Geometry check sheet. Reference: the model listing, model coordinates, mm. Face numbers are marked on the shaded views. Round coordinates to 2 decimals unless told otherwise and drop trailing zeros. Order: outer loops, then holes, each group sorted by start corner. A loop starts at its lowest first (then second) coordinate and runs counter-clockwise, first axis right, second up. Notation, with made-up numbers: (72, 70) - (89, 70) arc R12 ccw to (89, 81) - close; hole circle Ø2 at (-23.75, -5.5). An arc over 180 degrees is marked (long way). Write each question's results on one line, items separated by ' | '.
```python
from build123d import *

# Parameters (mm, degrees)
SKETCH1_W             = 17.78
SKETCH1_H             = 16.8148
BOSS_EXTRUDE1_DEPTH   = 3.175
SKETCH2_W             = 12.7
SKETCH2_H             = 4.7752
CUT_EXTRUDE1_DEPTH    = 13.64108776
F_8_CLEARANCE_HOLE1_D = 4.4958
F_0_CLEARANCE_HOLE1_D = 1.6129
F_1_72_TAPPED_HOLE1_D = 1.5113


with BuildPart() as part:
    # Sketch1 → Boss-Extrude1 (new body)
    with BuildSketch(Plane(origin=(0, 0, 0), x_dir=(1, 0, 0), z_dir=(0, 1, 0))):
        Rectangle(SKETCH1_W, SKETCH1_H)
    extrude(amount=BOSS_EXTRUDE1_DEPTH)

    # Sketch2 → Cut-Extrude1 (cut, through all)
    with BuildSketch(Plane(origin=(0, 3.175, 0), x_dir=(1, 0, 0), z_dir=(0, 1, 0))):
        with Locations((0, 8.4074)):
            Rectangle(SKETCH2_W, SKETCH2_H)
    extrude(amount=-CUT_EXTRUDE1_DEPTH, mode=Mode.SUBTRACT)

    # #8 Clearance Hole1 (through all)
    with Locations(Plane(origin=(0, 3.175, 0), x_dir=(1, 0, 0), z_dir=(0, 1, 0))):
        with Locations((0, -5.6134)):
            Hole(F_8_CLEARANCE_HOLE1_D / 2)

    # #0 Clearance Hole1 (through all)
    with Locations(Plane(origin=(8.89, 0, 0), x_dir=(0, 0, -1), z_dir=(1, 0, 0))):
        with Locations((7.2136, 1.5875)):
            Hole(F_0_CLEARANCE_HOLE1_D / 2)

    # #1-72 Tapped Hole1 (through all)
    with Locations(Plane(origin=(8.89, 0, 0), x_dir=(0, 0, -1), z_dir=(1, 0, 0))):
        with Locations((2.0574, 1.5875)):
            Hole(F_1_72_TAPPED_HOLE1_D / 2)


solid = part.part
```
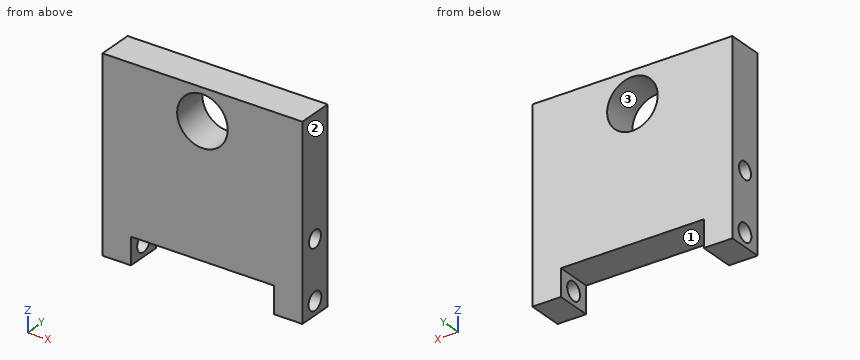
(1) Material ranges on line 1 (Z direction, x = 0, y = 1); line 2 (Z direction, x = 0, y = 1.1); line 3 (Z direction, x = -2.75, y = 2.7), recorded low to high.
Answers follow:
line 1: -6.02 to -2.53, -1.58 to 3.37, 7.86 to 8.41 | line 2: -6.02 to -2.63, -1.48 to 3.37, 7.86 to 8.41 | line 3: -6.02 to 8.41
(2) Depth check by flat-ended pin: pin 1 Ø1.5 at (y, z) = (1.59, -7.21) entering from -X (1 decimal); pin 2 Ø1 at (x, y) = (-0.5, 1.5) entering from -Z. Enter the tip coordinate at first touch or a pass-through.
Answers follow:
pin 1: through | pin 2: z = -6.02
(3) Section check C-C (z = 4). Record the cut outline in (x, y) (3 decimals), then the cut area to 3 significant figures.
Answers follow:
outline: (-8.89, 0) - (-1.565, 0) - (-1.565, 3.175) - (-8.89, 3.175) - close; (1.565, 0) - (8.89, 0) - (8.89, 3.175) - (1.565, 3.175) - close | area: 46.5 mm²
(4) Section check D-D (z = -6.75). Record the cut outline in (x, y) (3 decimals), then the cut area to 3 significant figures.
Answers follow:
outline: (-8.89, 0) - (-6.35, 0) - (-6.35, 0.928) - (-8.89, 0.928) - close; (-8.89, 2.247) - (-6.35, 2.247) - (-6.35, 3.175) - (-8.89, 3.175) - close; (6.35, 0) - (8.89, 0) - (8.89, 0.928) - (6.35, 0.928) - close; (6.35, 2.247) - (8.89, 2.247) - (8.89, 3.175) - (6.35, 3.175) - close | area: 9.42 mm²
(5) Draft check along Z on the marked faces 1, 2 and 3. Enter one of: released by +Z, released by -Z, zero draft, split by the parting line, or undercut.
Answers follow:
face 1: released by -Z | face 2: zero draft | face 3: undercut
(6) Section check B-B (y = 1.2). Record the cut outline in (x, z), then the cut area to 3 significant figures.
Answers follow:
outline: (-8.89, -8.41) - (-6.35, -8.41) - (-6.35, -7.92) - (-8.89, -7.92) - close; (-8.89, -6.51) - (-6.35, -6.51) - (-6.35, -6.02) - (6.35, -6.02) - (6.35, -6.51) - (8.89, -6.51) - (8.89, -2.71) - (-8.89, -2.71) - close; (-8.89, -1.41) - (8.89, -1.41) - (8.89, 8.41) - (-8.89, 8.41) - close; (6.35, -8.41) - (8.89, -8.41) - (8.89, -7.92) - (6.35, -7.92) - close; hole circle Ø4.5 at (0, 5.61) | area: 223 mm²
(7) Section check A-A (x = 0). Record the cut outline in (y, z) (1 decimal).
Answers follow:
outline: (0, -6) - (3.2, -6) - (3.2, 3.4) - (0, 3.4) - close; (0, 7.9) - (3.2, 7.9) - (3.2, 8.4) - (0, 8.4) - close; hole circle Ø1.5 at (1.6, -2.1)
